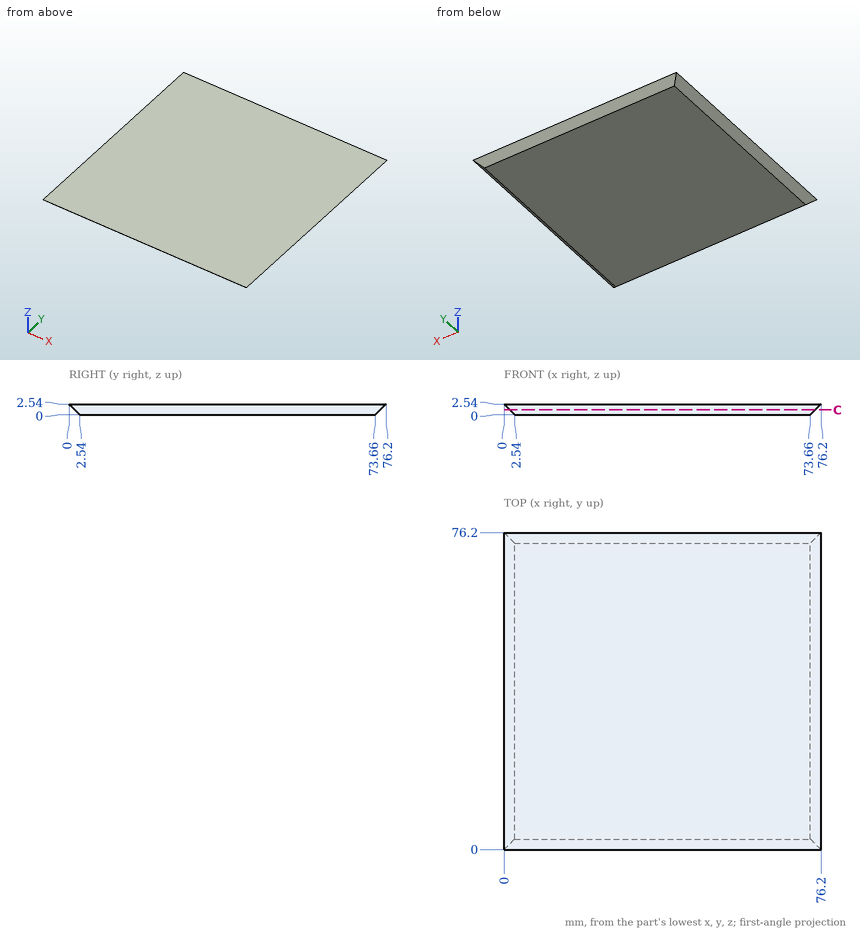
Input: dimensioned drawing with shaded views. Units: mm. Origin: part minimum x, y, z. Coordinates: 2 decimals unless noted, no trailing zeros. Write each loop counter-clockwise with the first axis right and the second up, starting at its lowest first coordinate (ties: lowest second). Pieces come first, ordered by that corner, then holes. Notation, with made-up numbers: (8, 21.5) -> (59, 21.5) arc R15 ccw to (59, 31.5) -> close; hole circle Ø7 at (0.25, 8). An arc over 180 degrees is marked (long way). Return JSON: item names as keys, results as strings. Group by question number.
1) Ray query, line 1 along X through (y, z) = (13, 1.5); line 2 along Y through (x, z) = (29.5, 1.3); line 3 along X through (y, z) = (63, 2.45). Return the intervals inside material, ascending.
2) Contact query for a flat-ended pin moving along its axis: P1, Ø1.5, axis at x = 66.5, z = 2, coming from the -Y side. Output: stop coordinate, or through.
3) Section query C-C, the plane z = 1.15. Return loops of the section in (x, y), plus the area to 3 significant figures.
From the geometry:
{
 "1": {"line 1": "1.04 to 75.16", "line 2": "1.24 to 74.96", "line 3": "0.09 to 76.11"},
 "2": {"P1": "y = 0"},
 "3": {"outline": "(1.39, 1.39) -> (74.81, 1.39) -> (74.81, 74.81) -> (1.39, 74.81) -> close", "area": "5,390 mm²"}
}
